from build123d import *

# Parameters (mm, degrees)
BOSS_EXTRUDE1_DEPTH = 800


with BuildPart() as part:
    # Sketch1 → Boss-Extrude1 (new body)
    with BuildSketch(Plane.XY):
        with BuildLine():
            Line((-185, 129.142135624), (-185, -129.142135624))
            Line((-185, -129.142135624), (-129.142135624, -185))
            Line((-129.142135624, -185), (-50, -185))
            Line((-50, -185), (-50, -175))
            ThreePointArc((-50, -175), (0, -125), (50, -175))
            Line((50, -175), (50, -185))
            Line((50, -185), (129.142135624, -185))
            Line((129.142135624, -185), (185, -129.142135624))
            Line((185, -129.142135624), (185, 129.142135624))
            Line((185, 129.142135624), (129.142135624, 185))
            Line((129.142135624, 185), (50, 185))
            Line((50, 185), (50, 175))
            ThreePointArc((50, 175), (0, 125), (-50, 175))
            Line((-50, 175), (-50, 185))
            Line((-50, 185), (-129.142135624, 185))
            Line((-129.142135624, 185), (-185, 129.142135624))
        make_face()
    extrude(amount=-BOSS_EXTRUDE1_DEPTH)


solid = part.part
Here's how the part is built. I have some questions about the finished solid (model axes, mm). Round coordinates to 2 decimals unless told otherwise and drop trailing zeros. Order: outer loops, then holes, each group sorted by start corner. A loop starts at its lowest first (then second) coordinate and runs counter-clockwise, first axis right, second up. Notation, with made-up numbers: M -9.75,-33.5 L 14.25,-33.5 A22 ccw 14.25,1.5 Z; hole C 61.25,-39 d9. An arc over 180 degrees is marked long. Return JSON: item names as keys, results as strings. Group by question number.
1. Please list where these lines run through material, in increasing order: probe 1 along X at (y, z) = (140.5, -275.5); probe 2 along X at (y, z) = (-131.5, -189); probe 3 along Y at (x, z) = (154, -330).
2. If we mould it in two halves opening along X, with no side actions, what happens to faces 1 (the face through (89, -185, -394)), 2 (the face through (-1.099, -125.012, -394.4)), 3 (the face through (185, -2, -394))? For each: pulls with the +X half, pulls with the -X half, needs draft (parallel to the pull), parting line crosses it, or undercut.
3. If we section it at B-B on x = 0: List the corners of the cut face in (y, z) for me, then the cut area to 3 significant figures.
4. If we section it at A-A on z = -303.5: List the corners of the cut face in (x, y) for me, then the cut area to 3 significant figures.
5. I'm going to push flat-ended pins straight in: pin 1 Ø5 at (y, z) = (-178.5, -342.5) entering from +X; pin 2 Ø10 at (x, z) = (-22, -349.5) entering from +Y; pin 3 Ø11 at (y, z) = (180.5, -312) entering from +X. Where does each tip first touch, or does it pass through?
Reply:
{
 "1": {"probe 1": "-173.64 to -36.19, 36.19 to 173.64", "probe 2": "-182.64 to -24.65, 24.65 to 182.64", "probe 3": "-160.14 to 160.14"},
 "2": {"face 1": "needs draft", "face 2": "undercut", "face 3": "pulls with the +X half"},
 "3": {"outline": "M -125,-800 L 125,-800 L 125,0 L -125,0 Z", "area": "200,000 mm^2"},
 "4": {"outline": "M -185,-129.14 L -129.14,-185 L -50,-185 L -50,-175 A50 cw 50,-175 L 50,-185 L 129.14,-185 L 185,-129.14 L 185,129.14 L 129.14,185 L 50,185 L 50,175 A50 cw -50,175 L -50,185 L -129.14,185 L -185,129.14 Z", "area": "121,000 mm^2"},
 "5": {"pin 1": "x = 138.14", "pin 2": "y = 132.92", "pin 3": "x = 139.14"}
}
